Check sheet for the drawn part. Datum: minimum x, y, z corner. Units: mm. Give positions to 0.01 mm unless a question says otherwise; leave off trailing zeros. Order: outer loops, then holes, each group sorted by start corner. A loop starts at its lowest first (then second) coordinate and runs counter-clockwise, first axis right, second up.
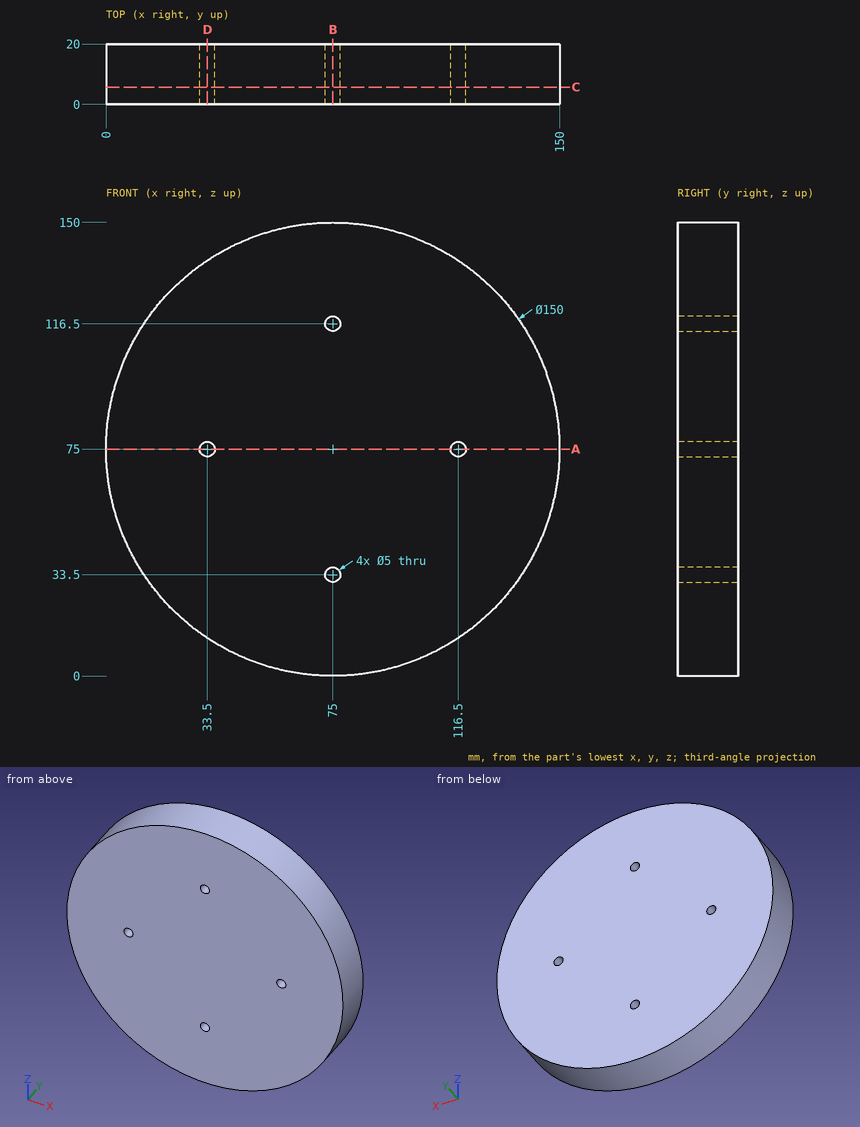
Q1. Go/stop test with flat-tipped pins: P1, Ø3, axis at x = 75, z = 116.5, coming from the +Y side; P2, Ø8, axis at x = 32, y = 13.5, coming from the -Z side; P3, Ø1.5, axis at y = 7, z = 122.5, coming from the +X side; P4, Ø10, axis at x = 64, y = 5.5, coming from the -Z side. Record where each tip stops, or that it passes through.
Q2. Sectioned sample at B-B, the plane x = 75. Record the cut outline in (y, z).
Q3. Sectioned sample at D-D, the plane x = 33.5. Record the cut outline in (y, z), plus the area to 3 significant figures.
Q4. Material ranges on line 1 (X direction, y = 4.5, z = 75); line 2 (X direction, y = 11.5, z = 116); line 3 (Z direction, x = 34.5, y = 19.25), recorded low to high.
Q5. Sectioned sample at A-A, the plane z = 75. Record the cut outline in (x, y), plus the area to 3 significant figures.
Q6. Sectioned sample at C-C, the plane y = 5.75. Record the cut outline in (x, z).
Filled in:
1. P1: passes through
1. P2: stops at z = 10.94
1. P3: stops at x = 133.65
1. P4: stops at z = 0.24
2. outline: (0, 0) - (20, 0) - (20, 31) - (0, 31) - close; (0, 36) - (20, 36) - (20, 114) - (0, 114) - close; (0, 119) - (20, 119) - (20, 150) - (0, 150) - close
3. outline: (0, 12.53) - (20, 12.53) - (20, 72.5) - (0, 72.5) - close; (0, 77.5) - (20, 77.5) - (20, 137.47) - (0, 137.47) - close
3. area: 2,400 mm2
4. line 1: x = 0 to 31, 36 to 114, 119 to 150
4. line 2: x = 12.2 to 72.55, 77.45 to 137.8
4. line 3: z = 11.88 to 72.71, 77.29 to 138.12
5. outline: (0, 0) - (31, 0) - (31, 20) - (0, 20) - close; (36, 0) - (114, 0) - (114, 20) - (36, 20) - close; (119, 0) - (150, 0) - (150, 20) - (119, 20) - close
5. area: 2,800 mm2
6. outline: circle Ø150 at (75, 75); hole circle Ø5 at (33.5, 75); hole circle Ø5 at (75, 33.5); hole circle Ø5 at (75, 116.5); hole circle Ø5 at (116.5, 75)
